from build123d import *

# Parameters (mm, degrees)
F1_DEPTH = 2.5
F2_DEPTH = 5


# Not quite as in the source:
# - a feature names something its author has since deleted; it is built from what else it names


with BuildPart() as f1:
    # F0 (on Front) → F1 (new body, symmetric)
    with BuildSketch(Plane.XZ):
        with BuildLine():
            ThreePointArc((39.686269666, -5), (39.9214903695, -2.5049165017), (40, 0))
            ThreePointArc((40, 0), (39.9214903695, 2.5049165017), (39.686269666, 5))
            ThreePointArc((39.686269666, 5), (28.2842712475, 28.2842712475), (5, 39.686269666))
            ThreePointArc((5, 39.686269666), (0, 40), (-5, 39.686269666))
            ThreePointArc((-5, 39.686269666), (-28.2842712475, 28.2842712475), (-39.686269666, 5))
            ThreePointArc((-39.686269666, 5), (-40, 0), (-39.686269666, -5))
            ThreePointArc((-39.686269666, -5), (-28.2842712475, -28.2842712475), (-5, -39.686269666))
            ThreePointArc((-5, -39.686269666), (0, -40), (5, -39.686269666))
            ThreePointArc((5, -39.686269666), (28.2842712475, -28.2842712475), (39.686269666, -5))
        make_face()
        with BuildLine():
            ThreePointArc((30.5941170816, 5), (30.8983626551, 2.5082235219), (31, 0))
            ThreePointArc((31, 0), (30.8983626551, -2.5082235219), (30.5941170816, -5))
            ThreePointArc((30.5941170816, -5), (21.9203102168, -21.9203102168), (5, -30.5941170816))
            ThreePointArc((5, -30.5941170816), (2.5082235219, -30.8983626551), (0, -31))
            ThreePointArc((0, -31), (-2.5082235219, -30.8983626551), (-5, -30.5941170816))
            ThreePointArc((-5, -30.5941170816), (-21.9203102168, -21.9203102168), (-30.5941170816, -5))
            ThreePointArc((-30.5941170816, -5), (-30.8983626551, -2.5082235219), (-31, 0))
            ThreePointArc((-31, 0), (-30.8983626551, 2.5082235219), (-30.5941170816, 5))
            ThreePointArc((-30.5941170816, 5), (-21.9203102168, 21.9203102168), (-5, 30.5941170816))
            ThreePointArc((-5, 30.5941170816), (-2.5082235219, 30.8983626551), (0, 31))
            ThreePointArc((0, 31), (2.5082235219, 30.8983626551), (5, 30.5941170816))
            ThreePointArc((5, 30.5941170816), (21.9203102168, 21.9203102168), (30.5941170816, 5))
        make_face(mode=Mode.SUBTRACT)
        with BuildLine():
            Line((7.5, 0), (31, 0))
            ThreePointArc((31, 0), (30.8983626551, 2.5082235219), (30.5941170816, 5))
            Line((30.5941170816, 5), (5.5901699437, 5))
            ThreePointArc((5.5901699437, 5), (7.0062926922, 2.6761656733), (7.5, 0))
        make_face()
        with BuildLine():
            ThreePointArc((30.5941170816, -5), (30.8983626551, -2.5082235219), (31, 0))
            Line((31, 0), (7.5, 0))
            ThreePointArc((7.5, 0), (7.0062926922, -2.6761656733), (5.5901699437, -5))
            Line((5.5901699437, -5), (30.5941170816, -5))
        make_face()
        with BuildLine():
            Line((2.5, 0), (7.5, 0))
            ThreePointArc((7.5, 0), (7.0062926922, 2.6761656733), (5.5901699437, 5))
            ThreePointArc((5.5901699437, 5), (5.3033008589, 5.3033008589), (5, 5.5901699437))
            ThreePointArc((5, 5.5901699437), (2.6761656733, 7.0062926922), (0, 7.5))
            Line((0, 7.5), (0, 2.5))
            ThreePointArc((0, 2.5), (1.767766953, 1.767766953), (2.5, 0))
        make_face()
        with BuildLine():
            ThreePointArc((5.5901699437, -5), (7.0062926922, -2.6761656733), (7.5, 0))
            Line((7.5, 0), (2.5, 0))
            ThreePointArc((2.5, 0), (1.767766953, -1.767766953), (0, -2.5))
            Line((0, -2.5), (0, -7.5))
            ThreePointArc((0, -7.5), (2.6761656733, -7.0062926922), (5, -5.5901699437))
            ThreePointArc((5, -5.5901699437), (5.3033008589, -5.3033008589), (5.5901699437, -5))
        make_face()
        with BuildLine():
            Line((5, 5.5901699437), (5, 30.5941170816))
            ThreePointArc((5, 30.5941170816), (2.5082235219, 30.8983626551), (0, 31))
            Line((0, 31), (0, 7.5))
            ThreePointArc((0, 7.5), (2.6761656733, 7.0062926922), (5, 5.5901699437))
        make_face()
        with BuildLine():
            ThreePointArc((0, -31), (2.5082235219, -30.8983626551), (5, -30.5941170816))
            Line((5, -30.5941170816), (5, -5.5901699437))
            ThreePointArc((5, -5.5901699437), (2.6761656733, -7.0062926922), (0, -7.5))
            Line((0, -7.5), (0, -31))
        make_face()
        with BuildLine():
            Line((0, 7.5), (0, 31))
            ThreePointArc((0, 31), (-2.5082235219, 30.8983626551), (-5, 30.5941170816))
            Line((-5, 30.5941170816), (-5, 5.5901699437))
            ThreePointArc((-5, 5.5901699437), (-2.6761656733, 7.0062926922), (0, 7.5))
        make_face()
        with BuildLine():
            ThreePointArc((-5, -30.5941170816), (-2.5082235219, -30.8983626551), (0, -31))
            Line((0, -31), (0, -7.5))
            ThreePointArc((0, -7.5), (-2.6761656733, -7.0062926922), (-5, -5.5901699437))
            Line((-5, -5.5901699437), (-5, -30.5941170816))
        make_face()
        with BuildLine():
            ThreePointArc((-2.5, 0), (-1.767766953, 1.767766953), (0, 2.5))
            Line((0, 2.5), (0, 7.5))
            ThreePointArc((0, 7.5), (-2.6761656733, 7.0062926922), (-5, 5.5901699437))
            ThreePointArc((-5, 5.5901699437), (-5.3033008589, 5.3033008589), (-5.5901699437, 5))
            ThreePointArc((-5.5901699437, 5), (-7.0062926922, 2.6761656733), (-7.5, 0))
            Line((-7.5, 0), (-2.5, 0))
        make_face()
        with BuildLine():
            Line((0, -7.5), (0, -2.5))
            ThreePointArc((0, -2.5), (-1.767766953, -1.767766953), (-2.5, 0))
            Line((-2.5, 0), (-7.5, 0))
            ThreePointArc((-7.5, 0), (-7.0062926922, -2.6761656733), (-5.5901699437, -5))
            ThreePointArc((-5.5901699437, -5), (-5.3033008589, -5.3033008589), (-5, -5.5901699437))
            ThreePointArc((-5, -5.5901699437), (-2.6761656733, -7.0062926922), (0, -7.5))
        make_face()
        with BuildLine():
            Line((-5.5901699437, 5), (-30.5941170816, 5))
            ThreePointArc((-30.5941170816, 5), (-30.8983626551, 2.5082235219), (-31, 0))
            Line((-31, 0), (-7.5, 0))
            ThreePointArc((-7.5, 0), (-7.0062926922, 2.6761656733), (-5.5901699437, 5))
        make_face()
        with BuildLine():
            ThreePointArc((-31, 0), (-30.8983626551, -2.5082235219), (-30.5941170816, -5))
            Line((-30.5941170816, -5), (-5.5901699437, -5))
            ThreePointArc((-5.5901699437, -5), (-7.0062926922, -2.6761656733), (-7.5, 0))
            Line((-7.5, 0), (-31, 0))
        make_face()
    extrude(amount=F1_DEPTH, both=True)

    # F2 (add): a face of the model
    f2_faces = [f1.faces().sort_by_distance(p)[0] for p in [
        (-38.5637724499, 2.5, 4.8585786438),
    ]]
    extrude(f2_faces, amount=F2_DEPTH)


solid = f1.part
Could you check a few things on this model? Use its own coordinates, in mm. Give positions to 0.01 mm unless a question says otherwise; leave off trailing zeros. Order: outer loops, then holes, each group sorted by start corner. A loop starts at its lowest first (then second) coordinate and runs counter-clockwise, first axis right, second up. Notation, with made-up numbers: (-32.75, -38) - (7.25, -38) arc R17 cw to (7.25, -30) - close; hole circle Ø7 at (72, 62). An arc over 180 degrees is marked (long way). Return JSON: item names as keys, results as strings. Group by question number.
Q1. Please list where these lines run through material, in increasing order: line 1 along Z through (x, y) = (-12.5, -0.25); line 2 along X through (y, z) = (1.5, -10); line 3 along Z through (x, y) = (24.5, 4.75). Write a range as [from, to].
Q2. Suppose I cut it at A-A, the plane y = 1.25. Please give me the cut outline in (x, z), and give its area (3 significant figures).
Q3. Suppose I cut it at B-B, the plane z = -21. Please give me the cut outline in (x, y).
Q4. Will these pins go through, and if not, where does the flat tip stop? pin 1 Ø4 at (y, z) = (-1.5, -13.5) entering from +X; pin 2 Ø2 at (x, y) = (-16.5, 0.5) entering from +Z; pin 3 Ø2 at (x, y) = (14, 1.5) entering from -Z; pin 4 Ø1.5 at (x, z) = (-6, -30) entering from +Y.
Q5. Suppose I cut it at C-C, the plane x = 22.5. Please give me the cut outline in (y, z).
Q6. Suppose I cut it at D-D, the plane x = 34. Please give me the cut outline in (y, z), and give its area (3 significant figures).
Resolved:
{
 "1": {"line 1": "z = [-38, -28.37], [-5, 5], [28.37, 38]", "line 2": "x = [-38.73, -29.34], [-5, 5], [29.34, 38.73]", "line 3": "z = [-31.62, -18.99], [-5, 5], [18.99, 31.62]"},
 "2": {"outline": "circle Ø80 at (0, 0); hole (-30.59, -5) arc R31 ccw to (-5, -30.59) - (-5, -5.59) arc R7.5 cw to (-5.59, -5) - close; hole (-30.59, 5) - (-5.59, 5) arc R7.5 cw to (-5, 5.59) - (-5, 30.59) arc R31 ccw to start; hole circle Ø5 at (0, 0); hole (5, -30.59) arc R31 ccw to (30.59, -5) - (5.59, -5) arc R7.5 cw to (5, -5.59) - close; hole (5, 5.59) arc R7.5 cw to (5.59, 5) - (30.59, 5) arc R31 ccw to (5, 30.59) - close", "area": "3,120 mm2"},
 "3": {"outline": "(-34.04, -2.5) - (-22.8, -2.5) - (-22.8, 7.5) - (-34.04, 7.5) - close; (-5, -2.5) - (5, -2.5) - (5, 7.5) - (-5, 7.5) - close; (22.8, -2.5) - (34.04, -2.5) - (34.04, 7.5) - (22.8, 7.5) - close"},
 "4": {"pin 1": "stops at x = 38.31", "pin 2": "stops at z = 36.87", "pin 3": "stops at z = -37.83", "pin 4": "stops at y = 7.5"},
 "5": {"outline": "(-2.5, -33.07) - (7.5, -33.07) - (7.5, -21.32) - (-2.5, -21.32) - close; (-2.5, -5) - (7.5, -5) - (7.5, 5) - (-2.5, 5) - close; (-2.5, 21.32) - (7.5, 21.32) - (7.5, 33.07) - (-2.5, 33.07) - close"},
 "6": {"outline": "(-2.5, -21.07) - (7.5, -21.07) - (7.5, 21.07) - (-2.5, 21.07) - close", "area": "421 mm2"}
}
